CAD build for the part. Positions are in the model's coordinates, mm. A direction names the side the tool comes from. Give positions to 0.01 mm unless a question says otherwise; leave off trailing zeros. Order: outer loops, then holes, each group sorted by start corner. A loop starts at its lowest first (then second) coordinate and runs counter-clockwise, first axis right, second up.
```python
from build123d import *

# Parameters (mm, degrees)
TAGLIO_ESTRUSIONE1_DEPTH    = 25.494897469
RIPETIZIONECIRCOLARE1_COUNT = 8


with BuildPart() as part:
    # Schizzo1 → Rivoluzione1 (revolve)
    with BuildSketch(Plane.XY, mode=Mode.PRIVATE) as rivoluzione1_sk:
        with BuildLine():
            Line((-18.601048223, 10), (-23.601048223, 10))
            Line((-23.601048223, 10), (-23.601048223, 3.5))
            Line((-23.601048223, 3.5), (-3.601048223, 3.5))
            Line((-3.601048223, 3.5), (-3.601048223, 4))
            ThreePointArc((-3.601048223, 4), (-3.893941442, 4.707106781), (-4.601048223, 5))
            Line((-4.601048223, 5), (-12.601048223, 5))
            Line((-12.601048223, 5), (-12.601048223, 9))
            ThreePointArc((-12.601048223, 9), (-12.893941442, 9.707106781), (-13.601048223, 10))
            Line((-13.601048223, 10), (-17.601048223, 10))
            Line((-17.601048223, 10), (-17.601048223, 6))
            Line((-17.601048223, 6), (-18.601048223, 6))
            Line((-18.601048223, 6), (-18.601048223, 10))
        make_face()
    revolve(rivoluzione1_sk.sketch.rotate(Axis((-39.30950846, 0, 0), (1, 0, 0)), 90), axis=Axis((-39.30950846, 0, 0), (1, 0, 0)))

    # Schizzo2 → Taglio-Estrusione1 (cut, through all)
    with BuildSketch(Plane.ZY.offset(23.601048223)):
        with BuildLine():
            Line((0.5, 4.974937186), (0.5, 10.752749152))
            Line((0.5, 10.752749152), (-0.5, 10.752749152))
            Line((-0.5, 10.752749152), (-0.5, 4.974937186))
            ThreePointArc((-0.5, 4.974937186), (0, 5), (0.5, 4.974937186))
        make_face()
    taglio_estrusione1 = extrude(amount=-TAGLIO_ESTRUSIONE1_DEPTH, mode=Mode.SUBTRACT)

    # RipetizioneCircolare1: Taglio-Estrusione1 ×8 about axis
    ripetizionecircolare1_axis = Axis((0, 0, 0), (1, 0, 0))
    for i in range(1, RIPETIZIONECIRCOLARE1_COUNT):
        add(taglio_estrusione1.rotate(ripetizionecircolare1_axis, i * 360 / RIPETIZIONECIRCOLARE1_COUNT), mode=Mode.SUBTRACT)


solid = part.part
```
Item 1: Two-plate mould, pull along Z, no slides. Class faces 4 (the face through (-15.63, 3.87, 9.22)), 5 (the face through (-19.4, 4.912, 5.619)), 6 (the face through (-17.601, -3, 7)): released by +Z, released by -Z, zero draft, split by the parting line, or undercut.
Item 2: Wall check: L1, parallel to Y at x = -19.5, z = 0; L2, parallel to X at y = 4.75, z = 7; L3, parallel to Z at x = -15.5, y = -6. Give the ranges that are in metal, low to high.
Item 3: Tool access for faces 1 (the face through (-19.4, -4.961, 5.668)), 2 (the face through (-19, 0.5, 8)), 3 (the face through (-18.108, -5.533, 2.32)): list every direction of +Z, -Z, +X, -X, +Y, -Y with a clear straight run to the whole face (end or side of a thin tool).
Item 4: Slice it at B-B (z = 0). Give the cut face in (x, y), and give its area (3 significant figures).
Item 5: Drop flat-ended pins along their axis: pin 1 Ø4 at (x, y) = (-20.5, -6.5) entering from +Z; pin 2 Ø4 at (x, y) = (-5.5, -6) entering from +Z; pin 3 Ø4.5 at (y, z) = (2.5, 8.5) entering from +X. Give the stop position or say it passes through.
A:
1. face 4: released by +Z
1. face 5: undercut
1. face 6: zero draft
2. L1: y = -5 to -3.5, 3.5 to 5
2. L2: x = -23.6 to -18.6, -17.6 to -12.6
2. L3: z = -8 to -6.71, -5.29 to -0.5, 0.5 to 5.29, 6.71 to 8
3. face 1: +X, -X
3. face 2: +Z, +X, -X
3. face 3: +Z, -Y
4. outline: (-23.6, -5) - (-4.6, -5) arc R1 ccw to (-3.6, -4) - (-3.6, -3.5) - (-23.6, -3.5) - close; (-23.6, 3.5) - (-3.6, 3.5) - (-3.6, 4) arc R1 ccw to (-4.6, 5) - (-23.6, 5) - close
4. area: 59.6 mm2
5. pin 1: stops at z = 8.93
5. pin 2: stops at z = 3
5. pin 3: stops at x = -12.6
